Could you check a few things on this drawing? It's one solid part, dimensions in mm from its lowest x, y, z. Give positions to 0.01 mm unless a question says otherwise; leave off trailing zeros. Order: outer loops, then holes, each group sorted by start corner. A loop starts at its lowest first (then second) coordinate and runs counter-clockwise, first axis right, second up. Notation, with made-up numbers: (22.25, -1.75) -> (43.25, -1.75) arc R13 ccw to (43.25, 14.25) -> close; hole circle Ø6 at (56, -3). An arc over 180 degrees is marked (long way). Answer as a JSON object with one key per item and string values.
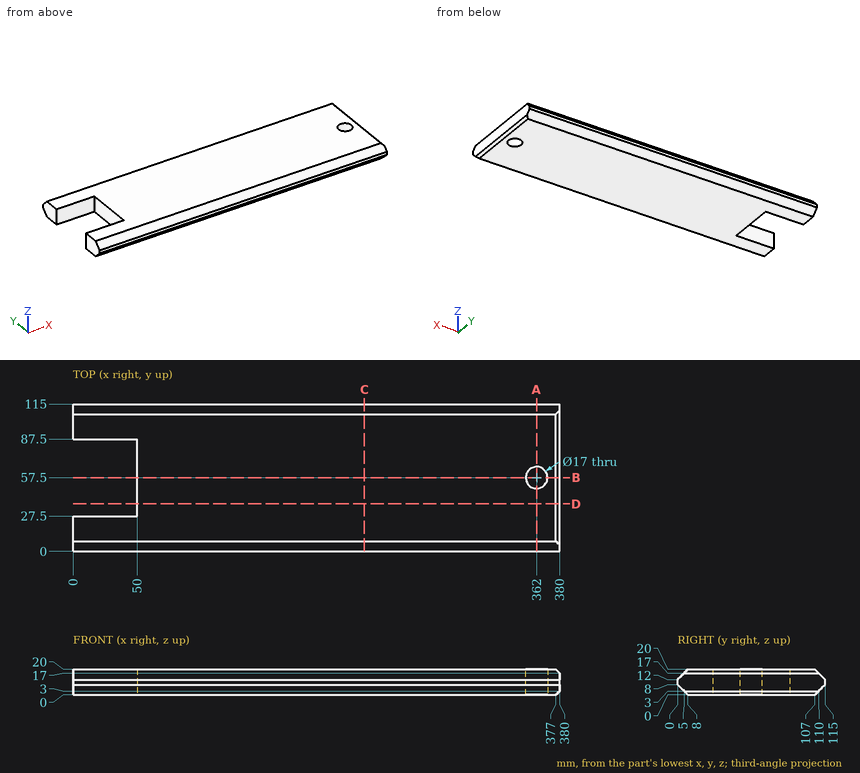
1. If we section it at B-B on y = 57.5: Please give me the cut outline in (x, z), then the cut area to 3 significant figures.
Worked answers:
{"outline": "(50, 0) -> (353.5, 0) -> (353.5, 20) -> (50, 20) -> close; (370.5, 0) -> (377, 0) -> (380, 3) -> (380, 17) -> (377, 20) -> (370.5, 20) -> close", "area": "6,250 mm²"}
2. If we section it at D-D on y = 37: Please give me the cut outline in (x, z).
Worked answers:
{"outline": "(50, 0) -> (377, 0) -> (380, 3) -> (380, 17) -> (377, 20) -> (50, 20) -> close"}
3. Will these pins go through, and if not, where does the flat tip stop? pin 1 Ø10 at (x, z) = (27, 14.5) entering from -Y; pin 2 Ø10 at (y, z) = (71.5, 15) entering from -X.
Worked answers:
{"pin 1": "y = 0", "pin 2": "x = 50"}
4. If we section it at C-C on x = 227.5: Please give me the cut outline in (y, z), then the cut area to 3 significant figures.
Worked answers:
{"outline": "(0, 8) -> (8, 0) -> (107, 0) -> (115, 8) -> (115, 12) -> (107, 20) -> (8, 20) -> (0, 12) -> close", "area": "2,170 mm²"}
5. If we section it at A-A on x = 362: Please give me the cut outline in (y, z), then the cut area to 3 significant figures.
Worked answers:
{"outline": "(0, 8) -> (8, 0) -> (49, 0) -> (49, 20) -> (8, 20) -> (0, 12) -> close; (66, 0) -> (107, 0) -> (115, 8) -> (115, 12) -> (107, 20) -> (66, 20) -> close", "area": "1,830 mm²"}
6. Please list where these lines run through material, in increasing order: L1, parallel to Y at x = 362, z = 8.5; L2, parallel to X at y = 72, z = 4.75; L3, parallel to Y at x = 362, z = 12.75.
Worked answers:
{"L1": "0 to 49, 66 to 115", "L2": "50 to 380", "L3": "0.75 to 49, 66 to 114.25"}
